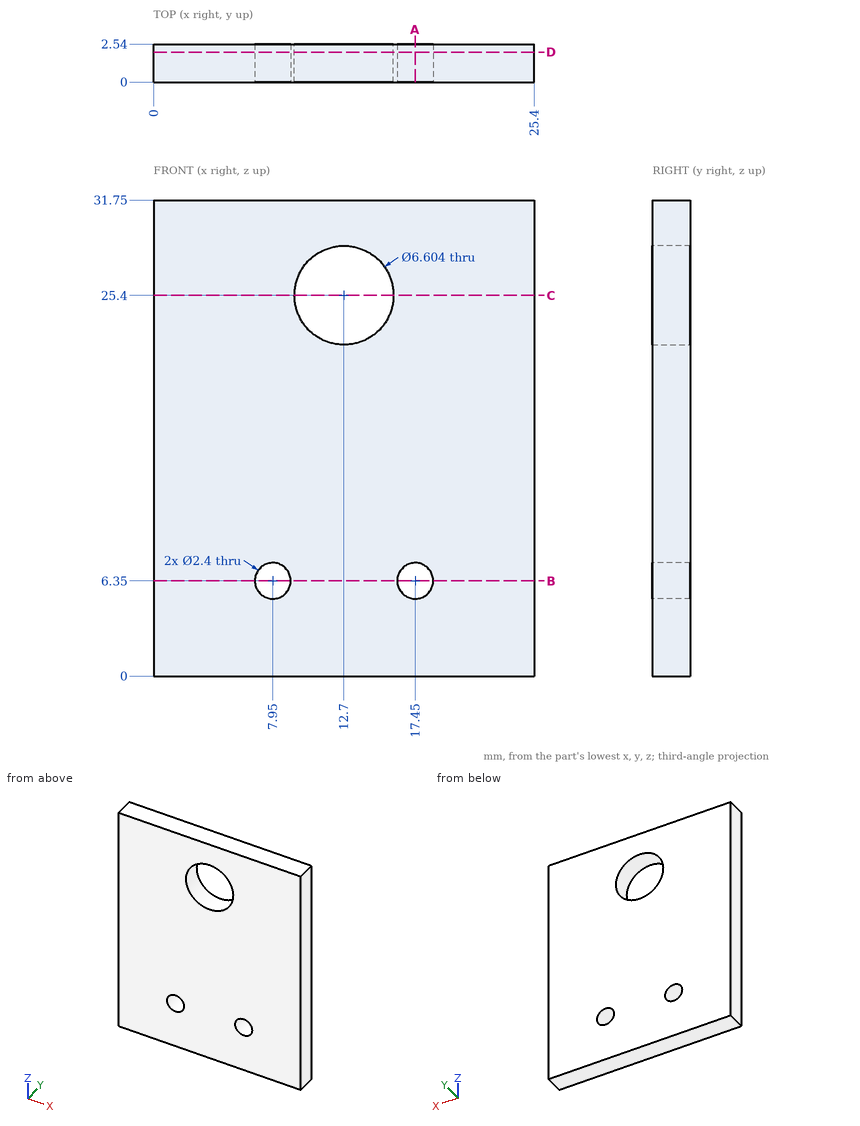
Check sheet for the drawn part. Datum: minimum x, y, z corner. Units: mm. Round coordinates to 2 decimals unless told otherwise and drop trailing zeros. Loops run counter-clockwise (first coordinate to the right, second up) from the corner with the lowest first, then second, coordinate; pieces in that order, holes last. Notation, with made-up numbers: (39.25, 60.25) - (53.25, 60.25) arc R3 cw to (53.25, 64.25) - close; hole circle Ø2 at (-1.75, -28). An arc over 180 degrees is marked (long way). Answer as a JSON object with one key per item and string values. Group by question number.
Q1. Sectioned sample at B-B, the plane z = 6.35. Enter the section's corners in (x, y), plus the area to 3 significant figures.
Q2. Scan lines: line 1 along Z through (x, y) = (7.95, 1.9); line 2 along X through (y, z) = (1.2, 6.5); line 3 along X through (y, z) = (0.7, 25.4). Record each from-to range of solid material in increasing order. Write a range as [from, to].
Q3. Sectioned sample at D-D, the plane y = 2. Enter the section's corners in (x, z).
Q4. Sectioned sample at A-A, the plane x = 17.45. Enter the section's corners in (y, z).
Q5. Gauge pin test, flat end, axial feed: P1, Ø10, axis at x = 22, z = 9.5, coming from the -Y side. Record the tip position at first contact, or that the pin passes through.
Q6. Sectioned sample at C-C, the plane z = 25.4. Enter the section's corners in (x, y).
Solution:
{
 "1": {"outline": "(0, 0) - (6.75, 0) - (6.75, 2.54) - (0, 2.54) - close; (9.15, 0) - (16.25, 0) - (16.25, 2.54) - (9.15, 2.54) - close; (18.65, 0) - (25.4, 0) - (25.4, 2.54) - (18.65, 2.54) - close", "area": "52.3 mm²"},
 "2": {"line 1": "z = [0, 5.15], [7.55, 31.75]", "line 2": "x = [0, 6.76], [9.14, 16.26], [18.64, 25.4]", "line 3": "x = [0, 9.4], [16, 25.4]"},
 "3": {"outline": "(0, 0) - (25.4, 0) - (25.4, 31.75) - (0, 31.75) - close; hole circle Ø2.4 at (7.95, 6.35); hole circle Ø6.6 at (12.7, 25.4); hole circle Ø2.4 at (17.45, 6.35)"},
 "4": {"outline": "(0, 0) - (2.54, 0) - (2.54, 5.15) - (0, 5.15) - close; (0, 7.55) - (2.54, 7.55) - (2.54, 31.75) - (0, 31.75) - close"},
 "5": {"P1": "stops at y = 0"},
 "6": {"outline": "(0, 0) - (9.4, 0) - (9.4, 2.54) - (0, 2.54) - close; (16, 0) - (25.4, 0) - (25.4, 2.54) - (16, 2.54) - close"}
}
